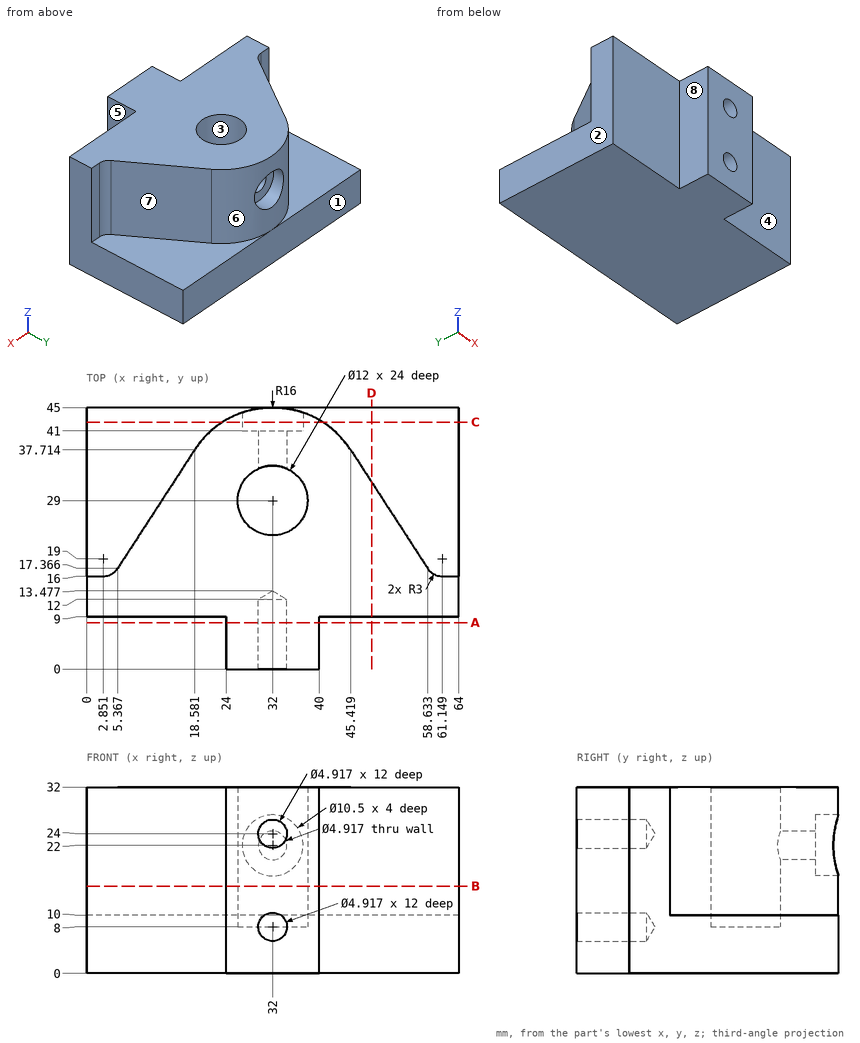
The drawing under review shows one solid part. Ordinate dimensions are in mm from its lowest x, y, z. A direction names the side the tool comes from. Round coordinates to 2 decimals unless told otherwise and drop trailing zeros. Write each loop counter-clockwise with the first axis right and the second up, starting at its lowest first coordinate (ties: lowest second). Pieces come first, ordered by that corner, then holes. Notation, with made-up numbers: (-7.75, -31.75) - (22.25, -31.75) arc R18 ccw to (22.25, -19.75) - close; hole circle Ø1 at (12, 23). An arc over 180 degrees is marked (long way). One line per question, with ' | ' between items.
Item 1: Add section B-B, the plane z = 15. Give the boundary of the cut face in (x, y).
Resolved:
outline: (0, 9) - (24, 9) - (24, 0) - (40, 0) - (40, 9) - (64, 9) - (64, 16) - (61.15, 16) arc R3 cw to (58.63, 17.37) - (45.42, 37.71) arc R16 ccw to (18.58, 37.71) - (5.37, 17.37) arc R3 cw to (2.85, 16) - (0, 16) - close; hole circle Ø12 at (32, 29)
Item 2: Add section A-A, the plane y = 8. Give the boundary of the cut face in (x, z).
Resolved:
outline: (24, 0) - (40, 0) - (40, 32) - (24, 32) - close; hole circle Ø4.92 at (32, 8); hole circle Ø4.92 at (32, 24)
Item 3: To check wall thickness, follow probe 1 along Z at (x, y) = (32, 2); probe 2 along X at (y, z) = (42.85, 22); probe 3 along Y at (x, z) = (32, 15.25). State the ranges of each line that lie inside material, in increasing order.
Resolved:
probe 1: z = 0 to 5.54, 10.46 to 21.54, 26.46 to 32 | probe 2: x = 23.99 to 26.75, 37.25 to 40.01 | probe 3: y = 0 to 23, 35 to 45
Item 4: Add section C-C, the plane y = 42.5. Give the boundary of the cut face in (x, z).
Resolved:
outline: (0, 0) - (64, 0) - (64, 10) - (40.59, 10) - (40.59, 32) - (23.41, 32) - (23.41, 10) - (0, 10) - close; hole circle Ø10.5 at (32, 22)
Item 5: For P1, Ø3, axis at x = 32, z = 24, coming from the +Y side; P2, Ø8.5, axis at x = 8.5, y = 34, coming from the +Z side; P3, Ø5, axis at y = 23, z = 22, coming from the -X side, all flat-tipped, find the tip position at first contact; note any pin that passes through.
Resolved:
P1: stops at y = 41 | P2: stops at z = 10 | P3: stops at x = 7.4
Item 6: Add section D-D, the plane x = 49. Give the boundary of the cut face in (y, z).
Resolved:
outline: (9, 0) - (45, 0) - (45, 10) - (32.2, 10) - (32.2, 32) - (9, 32) - close
Item 7: For the marked faces 5, 6, 7 and 8, list the 3-axis set-ups (+Z, -Z, +X, -X, +Y, -Y) from which the entire face can be reached by the end or side of a thin tool; tool diameter is ignored.
Resolved:
face 5: +Z, -Z, +X, -Y | face 6: +Z, +Y | face 7: +Z, +X, +Y | face 8: +Z, -Z, -X, -Y
Item 8: The part is to be moulded in two halves that separate along Y. For the marked faces 1, 2, 3 and 4, say which applies: pulls with the +Y half, pulls with the -Y half, needs draft (parallel to the pull), parting line crosses it, or undercut.
Resolved:
face 1: pulls with the +Y half | face 2: needs draft | face 3: undercut | face 4: pulls with the -Y half
